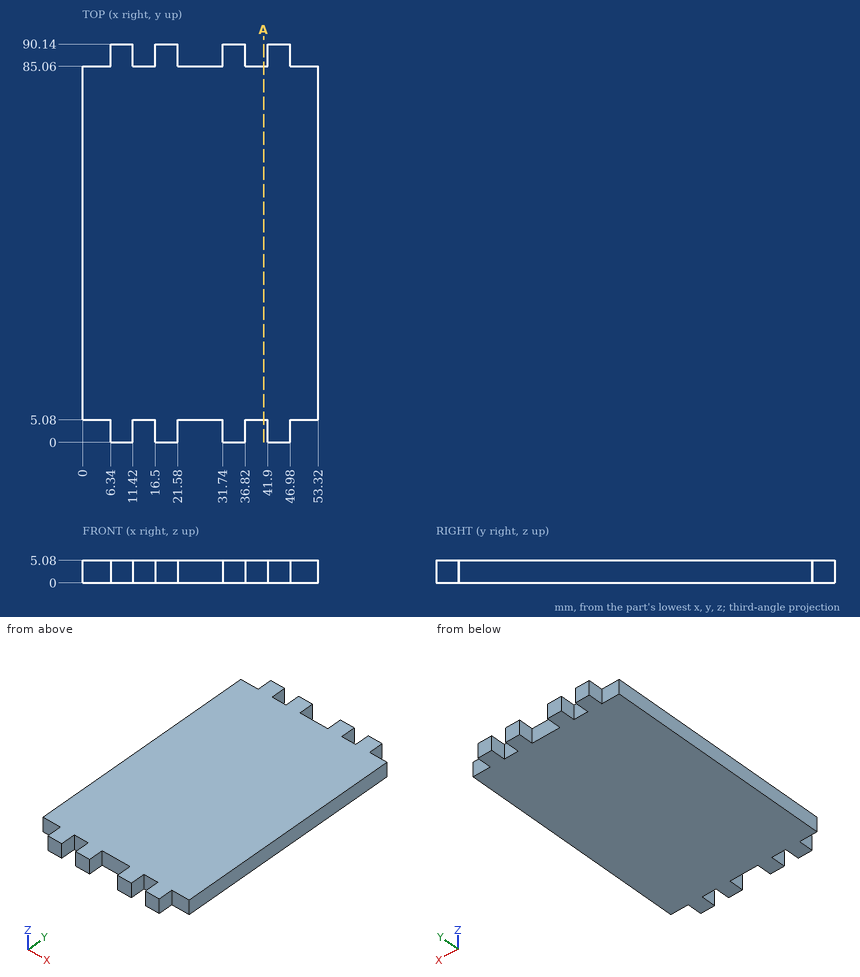
Drawing for the job (mm, zero at the part's lowest x, y, z). Give positions to 0.01 mm unless a question says otherwise; leave off trailing zeros. Order: outer loops, then holes, each group sorted by start corner. A loop starts at its lowest first (then second) coordinate and runs counter-clockwise, first axis right, second up. Notation, with made-up numbers: M 64,44.5 L 101,44.5 A33 cw 101,79.5 Z; hole C 79.25,-9 d8. An arc over 180 degrees is marked long. Put each result on its own line as item: value. Start each with the question number.
(1) Drill centre line: line 1 along Y through (x, z) = (28.5, 4.15). Where is it in solid material? Low to high.
(2) Flat gauge pins, fed straight in: pin 1 Ø1.5 at (x, z) = (49.5, 2) entering from +Y; pin 2 Ø1.5 at (x, z) = (14, 2) entering from -Y; pin 3 Ø1.5 at (y, z) = (87, 3) entering from +X. Where does each tip first touch, or does it go through?
(3) Saw through at A-A, the plane x = 41. Write the cut outline in (y, z), then the cut area to 3 significant figures.
Check result:
1. line 1: y = 5.08 to 85.06
2. pin 1: stops at y = 85.06
2. pin 2: stops at y = 5.08
2. pin 3: stops at x = 46.98
3. outline: M 5.08,0 L 85.06,0 L 85.06,5.08 L 5.08,5.08 Z
3. area: 406 mm2
